Read the model definition and answer for the solid it produces. Units are mm, in the model's axes. A direction names the side the tool comes from. Round coordinates to 2 decimals unless told otherwise and drop trailing zeros. Order: outer loops, then holes, each group sorted by start corner. A loop starts at its lowest first (then second) coordinate and runs counter-clockwise, first axis right, second up. Notation, with made-up numbers: (44, 29) -> (87, 29) arc R23 ccw to (87, 68) -> close; hole circle Ø11 at (-22.5, 86.25). An arc over 180 degrees is marked (long way). Use a Markdown table: item, result. Add a question column.
1. The mould has two halves that part along Z. Classify faces 3 (the face through (19.69, -5.53, 17.56)), 4 (the face through (3.895, -7.167, 1.592)), 5 (the face through (0, -3, 7)): +Z half, -Z half, draft (parallel to the pull), parting line (faces both ways), or undercut.
2. Given pin 1 (2 mm diameter, centred on x = 22.5, z = -7.5, fed in from -Y); pin 2 (6 mm diameter, centred on x = 20.5, y = -14.5, fed in from +Z); pin 3 (1.5 mm diameter, centred on y = -8, z = 10.5, fed in from +X), each flat-ended and moving along its own axis, determine where each tip first touches the part or whether it passes through.
3. Section B-B, the plane x = 23 is taken. Give the vertices of the cut face in (y, z).
4. Section A-A, the plane x = 19.5 is taken. Give the vertices of the cut face in (y, z).
5. For faces 1 (the face through (7.72, 7.71, -1.71)), 2 (the face through (3.219, -2.786, 8.848)), determine the directions among +Z, -Z, +X, -X, +Y, -Y from which every point of the face is accessible in a straight line to the end or side of a thin tool.
6. Consider L1, parallel to Y at x = 5, z = 0; L2, parallel to Z at x = 21.5, y = -9; L3, parallel to Z at x = 15, y = -2.5. Determine where each line is inside the solid, lowest interval first. Write a range as [from, to].
```python
from build123d import *

# Parameters (mm, degrees)
TAPPED_HOLE_FOR_9_16_12_HELICOIL1_D     = 14.68374
TAPPED_HOLE_FOR_9_16_12_HELICOIL1_DEPTH = 26.924
TAPPED_HOLE_FOR_9_16_12_HELICOIL1_TIP   = 4.411440553
FILLET1_R                               = 4.7625


with BuildPart() as part:
    # Sketch1 → Revolve1 (revolve)
    with BuildSketch(Plane.XY, mode=Mode.PRIVATE) as revolve1_sk:
        Polygon((0, 9.27608), (6.35, 9.27608), (7.662583372, 16.720110216), (32.815392318, 20.255106981), (32.815392318, 18.652005709), (9.025682257, 15.30858), (7.682070664, 7.68858), (7.682070664, 0), (0, 0), (0, 7.68858), align=None)
    revolve(revolve1_sk.sketch.rotate(Axis((0, 0, 0), (1, 0, 0)), 90), axis=Axis((0, 0, 0), (1, 0, 0)))

    # Tapped Hole for 9/16-12 Helicoil1
    with Locations(Plane.ZY):
        with Locations((0, 0)):
            Hole(TAPPED_HOLE_FOR_9_16_12_HELICOIL1_D / 2, depth=TAPPED_HOLE_FOR_9_16_12_HELICOIL1_DEPTH)
            with Locations((0, 0, -(TAPPED_HOLE_FOR_9_16_12_HELICOIL1_DEPTH + TAPPED_HOLE_FOR_9_16_12_HELICOIL1_TIP / 2))):  # 118° drill point
                Cone(0, TAPPED_HOLE_FOR_9_16_12_HELICOIL1_D / 2, TAPPED_HOLE_FOR_9_16_12_HELICOIL1_TIP, mode=Mode.SUBTRACT)

    # Fillet1
    fillet1_edges = [part.edges().sort_by_distance(p)[0] for p in [
        (9.025682257, 0, -15.30858),
        (7.662583372, 0, -16.720110216),
    ]]
    fillet(fillet1_edges, radius=FILLET1_R)


solid = part.part
```
Verdict:
| question | item | result |
|---|---|---|
| 1 | face 3 | parting line |
| 1 | face 4 | undercut |
| 1 | face 5 | draft |
| 2 | pin 1 | stops at y = -17.68 |
| 2 | pin 2 | stops at z = 14.58 |
| 2 | pin 3 | stops at x = 9.32 |
| 3 | outline | circle Ø37.75 at (0, 0); hole circle Ø34.55 at (0, 0) |
| 4 | outline | circle Ø36.77 at (0, 0); hole circle Ø33.56 at (0, 0) |
| 5 | face 1 | +X |
| 5 | face 2 | -X |
| 6 | L1 | y = [-9.28, -7.34], [7.34, 9.28] |
| 6 | L2 | z = [-16.35, -14.49], [14.49, 16.35] |
| 6 | L3 | z = [-17.57, -15.95], [15.95, 17.57] |
